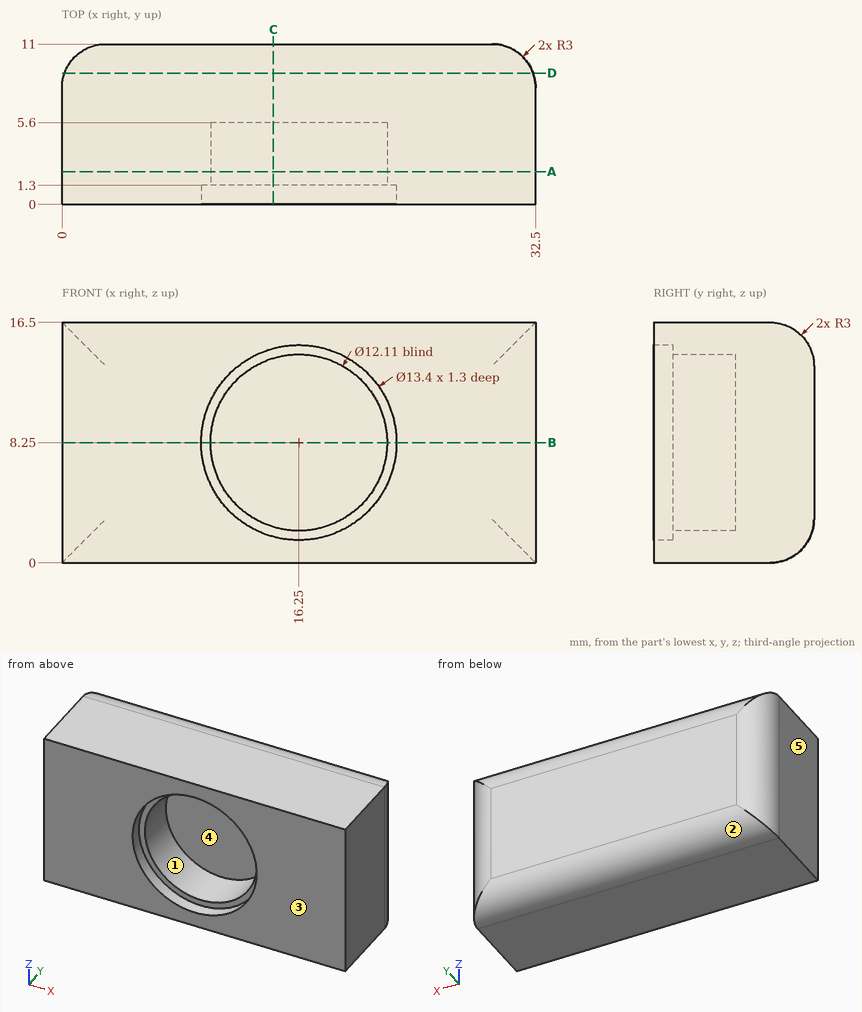
Answer from the drawing. Dimensions are ordinates in mm from the lowest x, y and z of the part. A direction names the side the tool comes from. Round coordinates to 2 decimals unless told otherwise and drop trailing zeros. Write each loop counter-clockwise with the first axis right and the second up, starting at its lowest first coordinate (ties: lowest second). Pieces come first, ordered by that corner, then holes.
1. Determine the mould class of the marked faces 1, 2 and 3 for opening direction Z: pulls with the +Z half, pulls with the -Z half, needs draft (parallel to the pull), parting line crosses it, or undercut.
2. The part is cut by section C-C, the plane x = 14.5. Determine the outline of the cut face in (y, z).
3. Given pin 1 Ø9.5 at (x, z) = (16.25, 8.25) entering from -Y, flat-ended and moving along its own axis, determine where the tip first touches the part or whether it passes through.
4. The part is cut by section D-D, the plane y = 9. Determine the outline of the cut face in (x, z), then the cut area to 3 significant figures.
5. The part is cut by section A-A, the plane y = 2.25. Determine the outline of the cut face in (x, z) (3 decimals), then the cut area to 3 significant figures.
6. Straight lines are drawn through the part: L1, parallel to X at y = 1.05, z = 8.25; L2, parallel to X at y = 3.3, z = 8.25 (3 decimals); L3, parallel to Y at x = 19, z = 13. For each, find the intervals that lie inside material, in ascending order.
7. Which of the six approach directions +Z, -Z, +X, -X, +Y, -Y give full straight-line access (tool end or side, diameter ignored) to the marked faces 4 and 5?
8. The part is cut by section B-B, the plane z = 8.25. Determine the outline of the cut face in (x, y) (3 decimals), then the cut area to 3 significant figures.
Values:
1. face 1: undercut
1. face 2: pulls with the -Z half
1. face 3: needs draft
2. outline: (0, 0) - (8, 0) arc R3 ccw to (11, 3) - (11, 13.5) arc R3 ccw to (8, 16.5) - (0, 16.5) - (0, 14.72) - (1.3, 14.72) - (1.3, 14.05) - (5.6, 14.05) - (5.6, 2.45) - (1.3, 2.45) - (1.3, 1.78) - (0, 1.78) - close
3. pin 1: stops at y = 5.6
4. outline: (0.17, 0.17) - (32.33, 0.17) - (32.33, 16.33) - (0.17, 16.33) - close
4. area: 520 mm2
5. outline: (0, 0) - (32.5, 0) - (32.5, 16.5) - (0, 16.5) - close; hole circle Ø12.11 at (16.25, 8.25)
5. area: 421 mm2
6. L1: x = 0 to 9.55, 22.95 to 32.5
6. L2: x = 0 to 10.195, 22.305 to 32.5
6. L3: y = 5.6 to 11
7. face 4: -Y
7. face 5: +Z, -Z, -X, +Y, -Y
8. outline: (0, 0) - (9.55, 0) - (9.55, 1.3) - (10.195, 1.3) - (10.195, 5.6) - (22.305, 5.6) - (22.305, 1.3) - (22.95, 1.3) - (22.95, 0) - (32.5, 0) - (32.5, 8) arc R3 ccw to (29.5, 11) - (3, 11) arc R3 ccw to (0, 8) - close
8. area: 284 mm2
